Answer from the drawing. Dimensions are ordinates in mm from the lowest x, y and z of the part. A direction names the side the tool comes from. Give positions to 0.01 mm unless a question says otherwise; leave off trailing zeros. Write each loop counter-clockwise with the first axis right and the second up, starting at its lowest first coordinate (ties: lowest second). Pieces come first, ordered by that corner, then holes. Notation, with made-up numbers: (81.5, -10.75) -> (139.5, -10.75) arc R13 cw to (139.5, -4.75) -> close; hole circle Ø3 at (69, 53.25). An arc over 180 degrees is marked (long way). Put each result on its own line as item: value. Start each with the question number.
1) Flat-ended cylindrical pins translate along their axes: pin 1 Ø1.5 at (y, z) = (14.5, 14) entering from -X; pin 2 Ø13 at (x, y) = (21.5, 14.5) entering from +Z; pin 3 Ø12 at (x, z) = (42, 14.5) entering from -Y (1 decimal). Find the tip coordinate at first contact, or state that the pin passes through.
2) A cutting plane is placed at D-D (z = 16). Write down the section's boundary in (x, y) (1 decimal), then the cut area to 3 significant figures.
3) Find the intervals of material crossed by line 1 along Z through (x, y) = (13, 24.5); line 2 along Y through (x, z) = (27.5, 71.5); line 3 along Y through (x, z) = (33, 44) (1 decimal), in increasing order. Write a range as from..to.
4) For a pull along X with two mould halves and no side action, classify the marked faces 3, 4 and 5 as released by +X, released by -X, zero draft, split by the parting line, or undercut.
5) A cutting plane is placed at C-C (y = 28.5). Write down the section's boundary in (x, z) (1 decimal), then the cut area to 3 significant figures.
6) For the marked faces 1 and 2, determine the directions among +Z, -Z, +X, -X, +Y, -Y from which every point of the face is accessible in a straight line to the end or side of a thin tool.
7) A cutting plane is placed at A-A (z = 68.5). Write down the section's boundary in (x, y) (1 decimal), then the cut area to 3 significant figures.
8) A cutting plane is placed at B-B (x = 13.5). Write down the section's boundary in (y, z) (1 decimal).
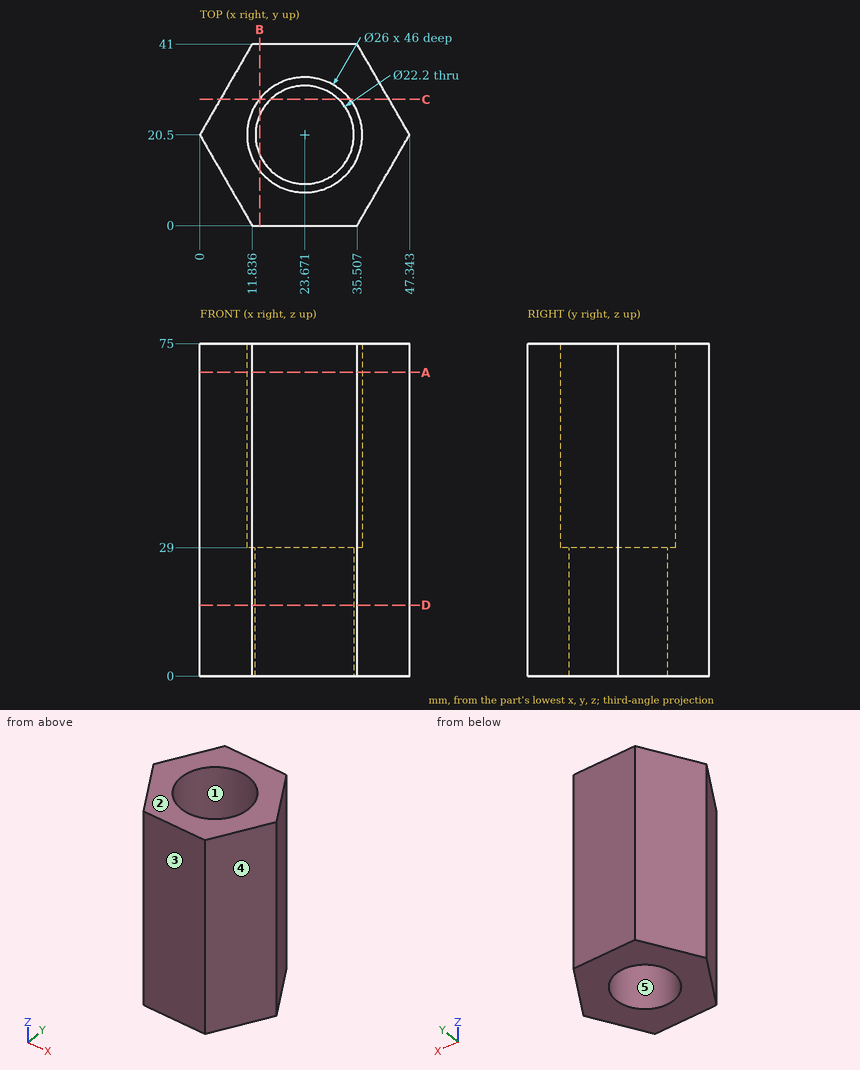
Reply:
1. pin 1: stops at x = 3.03
1. pin 2: stops at z = 29
1. pin 3: stops at y = 0.9
2. outline: (0, 20.5) -> (11.8, 0) -> (35.5, 0) -> (47.3, 20.5) -> (35.5, 41) -> (11.8, 41) -> close; hole circle Ø22.2 at (23.7, 20.5)
2. area: 1,070 mm2
3. line 1: z = 0..29
3. line 2: y = 0..8.08, 32.92..41
3. line 3: y = 0..11.4, 29.6..41
4. face 3: zero draft
4. face 4: released by +X
4. face 5: undercut
5. outline: (4.6, 0) -> (16, 0) -> (16, 29) -> (13.4, 29) -> (13.4, 75) -> (4.6, 75) -> close; (31.4, 0) -> (42.7, 0) -> (42.7, 75) -> (33.9, 75) -> (33.9, 29) -> (31.4, 29) -> close
5. area: 1,470 mm2
6. face 1: +Z
6. face 2: +Z, +X, -X, +Y, -Y
7. outline: (0, 20.5) -> (11.8, 0) -> (35.5, 0) -> (47.3, 20.5) -> (35.5, 41) -> (11.8, 41) -> close; hole circle Ø26 at (23.7, 20.5)
7. area: 925 mm2
8. outline: (0, 0) -> (16.1, 0) -> (16.1, 29) -> (12.4, 29) -> (12.4, 75) -> (0, 75) -> close; (24.9, 0) -> (41, 0) -> (41, 75) -> (28.6, 75) -> (28.6, 29) -> (24.9, 29) -> close
